```python
from build123d import *

# Parameters (mm, degrees)
SKETCH_2_W      = 240
SKETCH_2_H      = 20
SKETCH_2_R      = 2.1
EXTRUDE_1_DEPTH = 3
FILLET_1_R      = 3


with BuildPart() as part:
    # 草图2 → 凸台-拉伸1 (new body)
    with BuildSketch(Plane(origin=(0, 0, 0), x_dir=(1, 0, 0), z_dir=(0, 1, 0))):
        Rectangle(SKETCH_2_W, SKETCH_2_H)
        with Locations((-115, 5)):
            Circle(SKETCH_2_R, mode=Mode.SUBTRACT)
        with Locations((-95, 5)):
            Circle(SKETCH_2_R, mode=Mode.SUBTRACT)
        with Locations((-95, -5)):
            Circle(SKETCH_2_R, mode=Mode.SUBTRACT)
        with Locations((-115, -5)):
            Circle(SKETCH_2_R, mode=Mode.SUBTRACT)
        with Locations((115, -5)):
            Circle(SKETCH_2_R, mode=Mode.SUBTRACT)
        with Locations((95, -5)):
            Circle(SKETCH_2_R, mode=Mode.SUBTRACT)
        with Locations((95, 5)):
            Circle(SKETCH_2_R, mode=Mode.SUBTRACT)
        with Locations((115, 5)):
            Circle(SKETCH_2_R, mode=Mode.SUBTRACT)
    extrude(amount=EXTRUDE_1_DEPTH)

    # 圆角1
    fillet_1_edges = [part.edges().sort_by_distance(p)[0] for p in [
        (120, 1.5, 10),
        (-120, 1.5, 10),
        (-120, 1.5, -10),
        (120, 1.5, -10),
    ]]
    fillet(fillet_1_edges, radius=FILLET_1_R)


solid = part.part
```
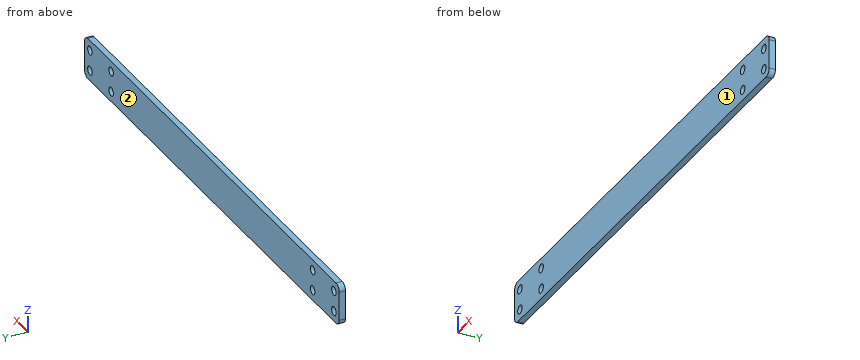
Part model, mm, in its own coordinate system. Face numbers are marked on the shaded views. Give positions to 0.01 mm unless a question says otherwise; leave off trailing zeros. Write each loop counter-clockwise with the first axis right and the second up, starting at its lowest first coordinate (ties: lowest second). Pieces come first, ordered by that corner, then holes. Notation, with made-up numbers: (-5.75, -9) -> (16.25, -9) arc R18 ccw to (16.25, 10) -> close; hole circle Ø11 at (-35, -14). An arc over 180 degrees is marked (long way). Put each result on its own line as item: value. Start each with the question number.
Item 1: Pin check, flat tip, straight feed: pin 1 Ø3.5 at (x, z) = (115, 5) entering from -Y. Stop position of the tip, or through.
Item 2: Cut at A-A (x = 115). List the corners of the cut face in (y, z).
Item 3: Cut at C-C (y = 1.6). State how many separate pieces and enclosed holes the cut face has, then the cut area to 3 significant figures.
Item 4: Wall check: L1, parallel to X at y = 0.65, z = 5; L2, parallel to Z at x = -95, y = 2.15; L3, parallel to X at y = 2.8, z = -4.5. Give the ranges that are in metal, low to high. Write a range as [from, to].
Item 5: Pull direction Y, two halves, no side cores. Call the marked faces 1 and 2: pulls with the +Y half, pulls with the -Y half, needs draft (parallel to the pull), parting line crosses it, or undercut.
Item 6: Cut at B-B (z = 5). List the corners of the cut face in (x, y).
Answer list:
1. pin 1: passes through
2. outline: (0, -10) -> (3, -10) -> (3, -7.1) -> (0, -7.1) -> close; (0, -2.9) -> (3, -2.9) -> (3, 2.9) -> (0, 2.9) -> close; (0, 7.1) -> (3, 7.1) -> (3, 10) -> (0, 10) -> close
3. separate pieces: 1
3. enclosed holes: 8
3. area: 4,680 mm2
4. L1: x = [-120, -117.1], [-112.9, -97.1], [-92.9, 92.9], [97.1, 112.9], [117.1, 120]
4. L2: z = [-10, -7.1], [-2.9, 2.9], [7.1, 10]
4. L3: x = [-120, -117.04], [-112.96, -97.04], [-92.96, 92.96], [97.04, 112.96], [117.04, 120]
5. face 1: pulls with the -Y half
5. face 2: pulls with the +Y half
6. outline: (-120, 0) -> (-117.1, 0) -> (-117.1, 3) -> (-120, 3) -> close; (-112.9, 0) -> (-97.1, 0) -> (-97.1, 3) -> (-112.9, 3) -> close; (-92.9, 0) -> (92.9, 0) -> (92.9, 3) -> (-92.9, 3) -> close; (97.1, 0) -> (112.9, 0) -> (112.9, 3) -> (97.1, 3) -> close; (117.1, 0) -> (120, 0) -> (120, 3) -> (117.1, 3) -> close
